from build123d import *

# Parameters (mm, degrees)
SKETCH1_R           = 16.75
BOSS_EXTRUDE1_DEPTH = 9
SKETCH2_R           = 15.125
BOSS_EXTRUDE2_DEPTH = 15.5
SKETCH3_R           = 3.5
BOSS_EXTRUDE3_DEPTH = 15.5
BOSS_EXTRUDE4_START = -15.5
SKETCH4_R           = 3.175
BOSS_EXTRUDE4_DEPTH = 28.5


with BuildPart() as part:
    # Sketch1 → Boss-Extrude1 (new body)
    with BuildSketch(Plane(origin=(0, 0, 0), x_dir=(1, 0, 0), z_dir=(0, 1, 0))):
        Circle(SKETCH1_R)
    extrude(amount=BOSS_EXTRUDE1_DEPTH)

    # Sketch2 → Boss-Extrude2 (add)
    with BuildSketch(Plane(origin=(0, 9, 0), x_dir=(1, 0, 0), z_dir=(0, 1, 0))):
        Circle(SKETCH2_R)
    extrude(amount=BOSS_EXTRUDE2_DEPTH)

    # Sketch3 → Boss-Extrude3 (add)
    with BuildSketch(Plane.XZ):
        with Locations((-12.5, 13.75)):
            Circle(SKETCH3_R)
        with Locations((12.5, 13.75)):
            Circle(SKETCH3_R)
        with Locations((12.5, -13.75)):
            Circle(SKETCH3_R)
        with Locations((-12.5, -13.75)):
            Circle(SKETCH3_R)
    extrude(amount=-BOSS_EXTRUDE3_DEPTH)

    # Sketch4 → Boss-Extrude4 (add)
    with BuildSketch(Plane(origin=(15.125, 0, 0), x_dir=(0, 0, -1), z_dir=(1, 0, 0)).offset(BOSS_EXTRUDE4_START)):
        with Locations((10.25, 15.5)):
            Circle(SKETCH4_R)
    boss_extrude4 = extrude(amount=BOSS_EXTRUDE4_DEPTH)

    # Mirror1: Boss-Extrude4 across plane
    add(boss_extrude4.mirror(Plane(origin=(0, 0, 0), x_dir=(0, 0, 1), z_dir=(1, 0, 0))))


solid = part.part
Read the model definition and answer for the solid it produces. Units are mm, in the model's axes. A direction names the side the tool comes from. Round coordinates to 2 decimals unless told otherwise and drop trailing zeros. Loops run counter-clockwise (first coordinate to the right, second up) from the corner with the lowest first, then second, coordinate; pieces in that order, holes last.
Q1. Which of the six approach directions +Z, -Z, +X, -X, +Y, -Y give full straight-line access (tool end or side, diameter ignored) to faces 3 (the face through (12, 15.5, -15)), 4 (the face through (-13, 15.5, -15)), 5 (the face through (-13, 15.5, 14))?
Q2. Section C-C on z = -9 is taken. Write down the section's boundary in (x, y) (3 decimals).
Q3. Each of these flat-tipped pins is pushed along its axis until it touches: pin 1 (8 mm diameter, centred on x = 17, y = 4.5, fed in from -Z); pin 2 (10 mm diameter, centred on y = 15, z = 5, fed in from -X) (3 decimals); pin 3 (1 mm diameter, centred on y = 3, z = -6.5, fed in from -X). Where does it stop, or does it pass through?
Q4. Section A-A on x = 0 is taken. Write down the section's boundary in (y, z) (3 decimals), and give its area (3 significant figures).
Q5. Consider probe 1 along Y at (x, z) = (10, 11.5); probe 2 along X at (y, z) = (7.25, 13.5); probe 3 along X at (y, z) = (3, 9). Determine where each line is inside the solid, lowest interval first.
Q6. Section D-D on x = 12.5 is taken. Write down the section's boundary in (y, z) (3 decimals).
Q7. Section B-B on y = 7.75 is taken. Write down the section's boundary in (x, z), and give its area (3 significant figures).
Q8. Determine the mould class of faces 1 (the face through (14.74, 7.64, -16.44)), 2 (the face through (-28.125, 16, -10)) for opening direction Z: released by +Z, released by -Z, zero draft, split by the parting line, or undercut.
Output:
1. face 3: -Z, +X, +Y
1. face 4: -Z, -X, +Y
1. face 5: +Z, -X, +Y
2. outline: (-28.125, 12.581) - (-12.156, 12.581) - (-12.156, 9) - (-14.127, 9) - (-14.127, 0) - (14.127, 0) - (14.127, 9) - (12.156, 9) - (12.156, 12.581) - (28.125, 12.581) - (28.125, 18.419) - (12.156, 18.419) - (12.156, 24.5) - (-12.156, 24.5) - (-12.156, 18.419) - (-28.125, 18.419) - close
3. pin 1: stops at z = -17.21
3. pin 2: stops at x = -15.125
3. pin 3: stops at x = -15.64
4. outline: (0, -16.75) - (9, -16.75) - (9, -15.125) - (24.5, -15.125) - (24.5, 15.125) - (9, 15.125) - (9, 16.75) - (0, 16.75) - close
4. area: 770 mm2
5. probe 1: y = 0 to 15.5
5. probe 2: x = -15.99 to 15.99
5. probe 3: x = -14.13 to 14.13
6. outline: (0, -17.25) - (15.5, -17.25) - (15.5, -13.425) arc R3.175 ccw to (18.159, -8.516) - (24.5, -8.516) - (24.5, 8.516) - (9, 8.516) - (9, 10.25) - (15.5, 10.25) - (15.5, 17.25) - (0, 17.25) - close; hole (9, -10.25) - (12.325, -10.25) arc R3.175 cw to (12.841, -8.516) - (9, -8.516) - close
7. outline: (-13.19, -10.32) arc R3.5 ccw (long way) to (-9.02, -14.11) arc R16.75 ccw to (9.02, -14.11) arc R3.5 ccw (long way) to (13.19, -10.32) arc R16.75 ccw to (13.19, 10.32) arc R3.5 ccw (long way) to (9.02, 14.11) arc R16.75 ccw to (-9.02, 14.11) arc R3.5 ccw (long way) to (-13.19, 10.32) arc R16.75 ccw to start
7. area: 1,010 mm2
8. face 1: undercut
8. face 2: zero draft
